CAD build for the part. Positions are in the model's coordinates, mm. A direction names the side the tool comes from. Coordinates: 2 decimals unless noted, no trailing zeros. Order: outer loops, then holes, each group sorted by start corner. A loop starts at its lowest first (then second) coordinate and runs counter-clockwise, first axis right, second up. Notation, with made-up numbers: (21.25, 31.5) - (40.25, 31.5) arc R18 cw to (40.25, 53.5) - close; hole circle Ø8 at (41.5, 28). An arc over 180 degrees is marked (long way). Use one line per item in the form item = value.
```python
from build123d import *

# Parameters (mm, degrees)
SKETCH1_W           = 108.5
SKETCH1_H           = 29.5
BOSS_EXTRUDE1_DEPTH = 2
SKETCH2_R           = 1.75
CUT_EXTRUDE1_DEPTH  = 3
FILLET1_R           = 3
SKETCH5_R           = 3.5
SKETCH5_W           = 14.5
SKETCH5_H           = 2.1
SKETCH5_W_2         = 2.75
SKETCH5_H_2         = 1
CUT_EXTRUDE2_DEPTH  = 3
FILLET2_R           = 0.2


with BuildPart() as part:
    # Sketch1 → Boss-Extrude1 (new body)
    with BuildSketch(Plane(origin=(0, 0, 0), x_dir=(1, 0, 0), z_dir=(0, 1, 0))):
        with Locations((54.25, 14.75)):
            Rectangle(SKETCH1_W, SKETCH1_H)
    extrude(amount=BOSS_EXTRUDE1_DEPTH)

    # Sketch2 → Cut-Extrude1 (cut, through all)
    with BuildSketch(Plane(origin=(0, 2, 0), x_dir=(1, 0, 0), z_dir=(0, 1, 0))):
        with Locations((6, 26.45)):
            Circle(SKETCH2_R)
        with Locations((6, 4.95)):
            Circle(SKETCH2_R)
        with Locations((102.5, 4.95)):
            Circle(SKETCH2_R)
        with Locations((102.5, 26.45)):
            Circle(SKETCH2_R)
    extrude(amount=-CUT_EXTRUDE1_DEPTH, mode=Mode.SUBTRACT)

    # Fillet1
    fillet1_edges = [part.edges().sort_by_distance(p)[0] for p in [
        (0, 1, -29.5),
        (108.5, 1, -29.5),
        (108.5, 1, 0),
        (0, 1, 0),
    ]]
    fillet(fillet1_edges, radius=FILLET1_R)

    # Sketch5 → Cut-Extrude2 (cut, through all)
    with BuildSketch(Plane(origin=(0, 2, 0), x_dir=(1, 0, 0), z_dir=(0, 1, 0))):
        with Locations((91.8, 11.9)):
            Circle(SKETCH5_R)
        with Locations((81, 11.9)):
            Circle(SKETCH5_R)
        with Locations((70.2, 11.9)):
            Circle(SKETCH5_R)
        with Locations((59.4, 11.9)):
            Circle(SKETCH5_R)
        with Locations((48.6, 11.9)):
            Circle(SKETCH5_R)
        with Locations((37.8, 11.9)):
            Circle(SKETCH5_R)
        with Locations((23.25, 21.15)):
            Rectangle(SKETCH5_W, SKETCH5_H)
        with Locations((17.475, 17.7)):
            Rectangle(SKETCH5_W_2, SKETCH5_H_2)
        with Locations((27.925, 17.7)):
            Rectangle(SKETCH5_W_2, SKETCH5_H_2)
    extrude(amount=-CUT_EXTRUDE2_DEPTH, mode=Mode.SUBTRACT)

    # Fillet2
    fillet2_edges = [part.edges().sort_by_distance(p)[0] for p in [
        (26.55, 1, -17.2),
        (26.55, 1, -18.2),
        (29.3, 1, -18.2),
        (29.3, 1, -17.2),
        (18.85, 1, -18.2),
        (18.85, 1, -17.2),
        (16.1, 1, -17.2),
        (16.1, 1, -18.2),
    ]]
    fillet(fillet2_edges, radius=FILLET2_R)


solid = part.part
```
Item 1: Two-plate mould, pull along Z, no slides. Class faces 1 (the face through (54, 1, -29.5)), 2 (the face through (5.62, 1.01, -3.24)), 3 (the face through (54, 1, 0)): +Z half, -Z half, draft (parallel to the pull), parting line (faces both ways), or undercut.
Derived:
face_1 = -Z half
face_2 = undercut
face_3 = +Z half
Item 2: Drill centre lines: line 1 (Z direction, x = 70.2, y = 1.5); line 2 (Z direction, x = 102.5, y = 1.5); line 3 (X direction, y = 0.9, z = -26.45). Where is each one in solid material? Low to high. Write a range as [from, to].
Derived:
line_1 = [-29.5, -15.4], [-8.4, 0]
line_2 = [-29.5, -28.2], [-24.7, -6.7], [-3.2, 0]
line_3 = [0, 4.25], [7.75, 100.75], [104.25, 108.5]
Item 3: Cut at D-D, the plane y = 1.25. State how many separate pieces and enclosed holes the cut face has, plus the area to 3 significant figures.
Derived:
separate_pieces = 1
enclosed_holes = 13
area = 2,890 mm²
Item 4: Cut at A-A, the plane x = 102.5. Write the cut outline in (y, z), plus the area to 3 significant figures.
Derived:
outline = (0, -29.5) - (2, -29.5) - (2, -28.2) - (0, -28.2) - close; (0, -24.7) - (2, -24.7) - (2, -6.7) - (0, -6.7) - close; (0, -3.2) - (2, -3.2) - (2, 0) - (0, 0) - close
area = 45.0 mm²
Item 5: 3-axis set-ups, long thin cutter, end or side, ignore diameter. For faces 4 (the face through (23, 1, -22.2)), 5 (the face through (0, 1, -15)): which of +Z, -Z, +X, -X, +Y, -Y reach the whole face in a straight line?
Derived:
face_4 = +Y, -Y
face_5 = +Z, -Z, -X, +Y, -Y
Item 6: Cut at B-B, the plane z = -11.9. Write the cut outline in (x, y), plus the area to 3 significant figures.
Derived:
outline = (0, 0) - (34.3, 0) - (34.3, 2) - (0, 2) - close; (41.3, 0) - (45.1, 0) - (45.1, 2) - (41.3, 2) - close; (52.1, 0) - (55.9, 0) - (55.9, 2) - (52.1, 2) - close; (62.9, 0) - (66.7, 0) - (66.7, 2) - (62.9, 2) - close; (73.7, 0) - (77.5, 0) - (77.5, 2) - (73.7, 2) - close; (84.5, 0) - (88.3, 0) - (88.3, 2) - (84.5, 2) - close; (95.3, 0) - (108.5, 0) - (108.5, 2) - (95.3, 2) - close
area = 133 mm²
Item 7: Drop flat-ended pins along their axis: pin 1 (4 mm diameter, centred on x = 102.5, z = -4.95, fed in from +Y); pin 2 (4 mm diameter, centred on x = 91.8, z = -11.9, fed in from +Y). Give the stop position or say it passes through.
Derived:
pin_1 = 2
pin_2 = through
Item 8: Cut at C-C, the plane x = 59.4. Write the cut outline in (y, z).
Derived:
outline = (0, -29.5) - (2, -29.5) - (2, -15.4) - (0, -15.4) - close; (0, -8.4) - (2, -8.4) - (2, 0) - (0, 0) - close
